Could you check a few things on this drawing? It's one solid part, dimensions in mm from its lowest x, y, z. Round coordinates to 2 decimals unless told otherwise and drop trailing zeros. Order: outer loops, then holes, each group sorted by start corner. A loop starts at its lowest first (then second) coordinate and runs counter-clockwise, first axis right, second up. Notation, with made-up numbers: M 9.25,44 L 19.25,44 A13 cw 19.25,54 Z; hole C -2,69.5 d1. An arc over 180 degrees is marked long. Answer as CSV lines item,"result". Start each with the question number.
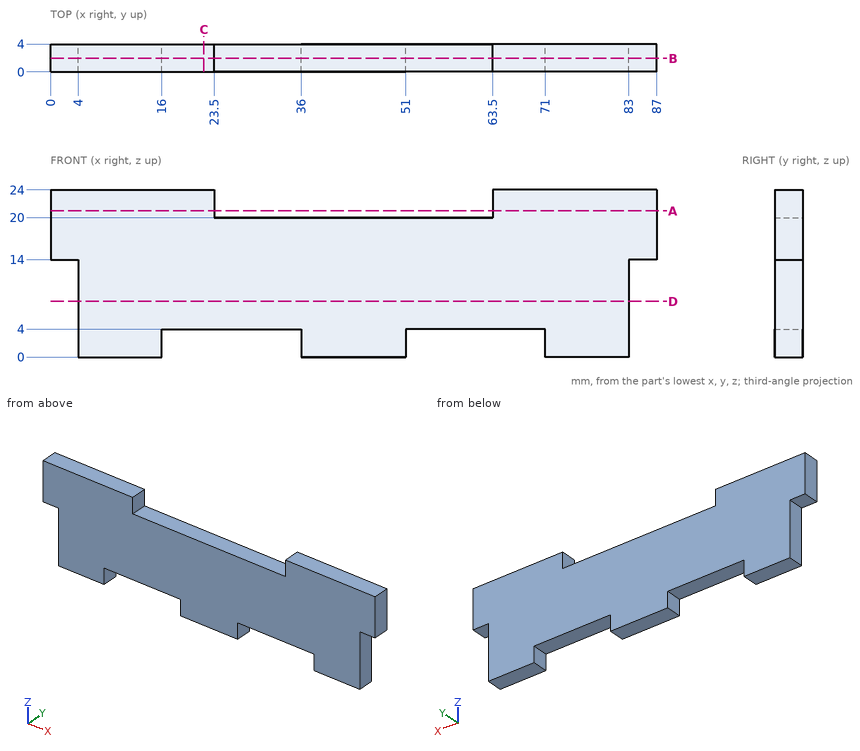
Item 1: If we section it at C-C on x = 22: Please give me the cut outline in (y, z), and give its area (3 significant figures).
Item 2: If we section it at B-B on y = 1.95: Please give me the cut outline in (x, z), and give its area (3 significant figures).
Item 3: If we section it at D-D on z = 8: Please give me the cut outline in (x, y), and give its area (3 significant figures).
Item 4: If I drill on line 1 along X through (y, z) = (1.65, 1.75); line 2 along X through (y, z) = (2.8, 22); line 3 along Z through (x, y) = (35, 3.3), over which ranges is the centre line in solid material (lowest first)?
Item 5: If we section it at A-A on z = 21: Please give me the cut outline in (x, y), and give its area (3 significant figures).
Item 6: For P1, Ø1.5, axis at y = 2, z = 13.5, coming from the +X side; P2, Ø2, axis at x = 85, y = 2, coming from the -Z side; P3, Ø1.2, axis at y = 2.5, z = 2.5, coming from the +X side; P4, Ø2, axis at y = 2.5, z = 9, coming from the -X side, each with a flat end and sliding along its axis, tell me the tip position at first contact or that it passes through.
Geometry says:
1,outline,"M 0,4 L 4,4 L 4,24 L 0,24 Z"
1,area,"80.0 mm²"
2,outline,"M 0,14 L 4,14 L 4,0 L 16,0 L 16,4 L 36,4 L 36,0 L 51,0 L 51,4 L 71,4 L 71,0 L 83,0 L 83,14 L 87,14 L 87,24 L 63.5,24 L 63.5,20 L 23.5,20 L 23.5,24 L 0,24 Z"
2,area,"1,660 mm²"
3,outline,"M 4,0 L 83,0 L 83,4 L 4,4 Z"
3,area,"316 mm²"
4,line 1,"4 to 16, 36 to 51, 71 to 83"
4,line 2,"0 to 23.5, 63.5 to 87"
4,line 3,"4 to 20"
5,outline,"M 0,0 L 23.5,0 L 23.5,4 L 0,4 Z; M 63.5,0 L 87,0 L 87,4 L 63.5,4 Z"
5,area,"188 mm²"
6,P1,"x = 87"
6,P2,"z = 14"
6,P3,"x = 83"
6,P4,"x = 4"
